Design review of the part built by this model. Coordinates are the model's own, in mm. A direction names the side the tool comes from. Round coordinates to 2 decimals unless told otherwise and drop trailing zeros. Write each loop counter-clockwise with the first axis right and the second up, starting at its lowest first coordinate (ties: lowest second). Pieces come first, ordered by that corner, then holes. Notation, with made-up numbers: M 16.5,-36.5 L 36.5,-36.5 A22 cw 36.5,-19.5 Z; hole C 12,22 d4. An arc over 180 degrees is marked long. One line per question, with ' | ' between items. Start each with the question number.
Item 1: Add section C-C, the plane y = 22.5. State the section outline as (x, z) points (3 decimals), and give its area (3 significant figures).
Item 2: Insertion check: pin 1 Ø6 at (y, z) = (35, 81) entering from -X (3 decimals); pin 2 Ø3 at (x, y) = (17.5, -11) entering from -Z; pin 3 Ø3 at (y, z) = (4.5, 4) entering from -X (3 decimals); pin 4 Ø4 at (x, z) = (96, 188.5) entering from +Y (3 decimals). Each pin has a flat end and moves straight along its axis. Give the tip position at first contact, or say it passes through.
Item 3: Draft analysis for pull direction Z (two halves, no side actions). For faces 5 (the face through (-4, -2, 82.55)), 6 (the face through (-4, -9.525, 251)), 7 (the face through (-2, 1, 0)), 8 (the face through (-48.317, 31.527, 170.739)), state which applies: released by +Z, released by -Z, zero draft, split by the parting line, or undercut.
Item 4: For L1, parallel to Z at x = 95, y = -74; L2, parallel to Y at x = -180.5, z = 269 (3 decimals); L3, parallel to Y at x = -31.5, z = 218 (3 decimals), list the stretches that pass through material, from the lowest coordinate up.
Item 5: Add section D-D, the plane x = 32.5. State the section outline as (y, z) points (3 decimals).
Item 6: Machinability: for faces 1 (the face through (-15.875, 36, 63)), 2 (the face through (-11.891, 20.076, 62.7)), 3 (the face through (11.674, 19.859, 62.7)), 4 (the face through (49.438, 30.884, 170.739)), which of the approach directions +Z, -Z, +X, -X, +Y, -Y give a long, thin tool a straight path to every point of the face, cutting with its end or side? Answer none if there is none.
Item 7: Add section B-B, the plane x = 146. State the section outline as (y, z) points (3 decimals).
Item 8: Add section A-A, the plane z = 171. State the section outline as (x, y) points (3 decimals), and give its area (3 significant figures).
```python
from build123d import *

# Parameters (mm, degrees)
F1_DEPTH = 6.35
F3_DEPTH = 114.3
F5_DEPTH = 101.6
F7_DEPTH = 20.32
F8_W     = 527.05
F8_H     = 295.275
F9_DEPTH = 2.54


with BuildPart() as f1:
    # F0 (on Top) → F1 (new body)
    with BuildSketch(Plane.XY):
        with BuildLine():
            Line((-114.3, -98.425), (114.3, -98.425))
            ThreePointArc((114.3, -98.425), (121.0351920908, -95.6351920908), (123.825, -88.9))
            Line((123.825, -88.9), (123.825, 88.9))
            ThreePointArc((123.825, 88.9), (121.0351920908, 95.6351920908), (114.3, 98.425))
            Line((114.3, 98.425), (-114.3, 98.425))
            ThreePointArc((-114.3, 98.425), (-121.0351920908, 95.6351920908), (-123.825, 88.9))
            Line((-123.825, 88.9), (-123.825, -88.9))
            ThreePointArc((-123.825, -88.9), (-121.0351920908, -95.6351920908), (-114.3, -98.425))
        make_face()
    extrude(amount=F1_DEPTH)

    # F2 (on face) → F3 (join)
    with BuildSketch(Plane.XY.offset(6.35)):
        with BuildLine():
            Line((-1.905, 15.875), (1.905, 15.875))
            ThreePointArc((1.905, 15.875), (11.7832817332, 19.9667182668), (15.875, 29.845))
            Line((15.875, 29.845), (15.875, 42.037))
            ThreePointArc((15.875, 42.037), (11.7832817332, 51.9152817332), (1.905, 56.007))
            Line((1.905, 56.007), (-1.905, 56.007))
            ThreePointArc((-1.905, 56.007), (-11.7832817332, 51.9152817332), (-15.875, 42.037))
            Line((-15.875, 42.037), (-15.875, 29.845))
            ThreePointArc((-15.875, 29.845), (-11.7832817332, 19.9667182668), (-1.905, 15.875))
        make_face()
    extrude(amount=F3_DEPTH)

    # F4 (on face) → F5 (join)
    with BuildSketch(Plane.XY.offset(120.65)):
        with BuildLine():
            ThreePointArc((-15.875, 42.037), (-13.9930859093, 49.0397908043), (-8.8543730782, 54.1558742802))
            Line((-8.8543730782, 54.1558742802), (-88.9, 8.255))
            Line((-88.9, 8.255), (88.9, 8.255))
            Line((88.9, 8.255), (8.8543730782, 54.1558742802))
            ThreePointArc((8.8543730782, 54.1558742802), (13.9930859093, 49.0397908043), (15.875, 42.037))
            Line((15.875, 42.037), (15.875, 29.845))
            ThreePointArc((15.875, 29.845), (11.7832817332, 19.9667182668), (1.905, 15.875))
            Line((1.905, 15.875), (-1.905, 15.875))
            ThreePointArc((-1.905, 15.875), (-11.7832817332, 19.9667182668), (-15.875, 29.845))
            Line((-15.875, 29.845), (-15.875, 42.037))
        make_face()
        with BuildLine():
            ThreePointArc((-1.905, 56.007), (-5.5008466531, 55.536288383), (-8.8543730782, 54.1558742802))
            ThreePointArc((-8.8543730782, 54.1558742802), (-13.9930859093, 49.0397908043), (-15.875, 42.037))
            Line((-15.875, 42.037), (-15.875, 29.845))
            ThreePointArc((-15.875, 29.845), (-11.7832817332, 19.9667182668), (-1.905, 15.875))
            Line((-1.905, 15.875), (1.905, 15.875))
            ThreePointArc((1.905, 15.875), (11.7832817332, 19.9667182668), (15.875, 29.845))
            Line((15.875, 29.845), (15.875, 42.037))
            ThreePointArc((15.875, 42.037), (13.9930859093, 49.0397908043), (8.8543730782, 54.1558742802))
            ThreePointArc((8.8543730782, 54.1558742802), (5.5008466531, 55.536288383), (1.905, 56.007))
            Line((1.905, 56.007), (-1.905, 56.007))
        make_face()
    extrude(amount=F5_DEPTH)

    # F6 (on face) → F7 (join)
    with BuildSketch(Plane.XZ.offset(-8.255)):
        with BuildLine():
            Line((263.525, 406.4), (-263.525, 406.4))
            ThreePointArc((-263.525, 406.4), (-270.2601920908, 403.6101920908), (-273.05, 396.875))
            Line((-273.05, 396.875), (-273.05, 92.075))
            ThreePointArc((-273.05, 92.075), (-270.2601920908, 85.3398079092), (-263.525, 82.55))
            Line((-263.525, 82.55), (263.525, 82.55))
            ThreePointArc((263.525, 82.55), (270.2601920908, 85.3398079092), (273.05, 92.075))
            Line((273.05, 92.075), (273.05, 396.875))
            ThreePointArc((273.05, 396.875), (270.2601920908, 403.6101920908), (263.525, 406.4))
        make_face()
    extrude(amount=F7_DEPTH)

    # F8 (on face) → F9 (cut)
    with BuildSketch(Plane.XZ.offset(12.065)):
        with Locations((0, 249.2375)):
            Rectangle(F8_W, F8_H)
    extrude(amount=-F9_DEPTH, mode=Mode.SUBTRACT)


solid = f1.part
```
Computed values:
1) outline: M -123.825,0 L 123.825,0 L 123.825,6.35 L 13.788,6.35 L 13.788,120.65 L 64.058,120.65 L 64.058,222.25 L -64.058,222.25 L -64.058,120.65 L -13.788,120.65 L -13.788,6.35 L -123.825,6.35 Z | area: 17,700 mm^2
2) pin 1: stops at x = -15.875 | pin 2: stops at z = 0 | pin 3: stops at x = -123.825 | pin 4: stops at y = 8.255
3) face 5: undercut | face 6: undercut | face 7: released by -Z | face 8: zero draft
4) L1: z = 0 to 6.35 | L2: y = -9.525 to 8.255 | L3: y = -9.525 to 41.17
5) outline: M -98.425,0 L 98.425,0 L 98.425,6.35 L -98.425,6.35 Z; M -12.065,82.55 L 8.255,82.55 L 8.255,120.65 L 40.597,120.65 L 40.597,222.25 L 8.255,222.25 L 8.255,406.4 L -12.065,406.4 L -12.065,396.875 L -9.525,396.875 L -9.525,101.6 L -12.065,101.6 Z
6) face 1: -X, +Y | face 2: -X | face 3: +X | face 4: +Z, +X, +Y
7) outline: M -12.065,82.55 L 8.255,82.55 L 8.255,406.4 L -12.065,406.4 L -12.065,396.875 L -9.525,396.875 L -9.525,101.6 L -12.065,101.6 Z
8) outline: M -273.05,-12.065 L -263.525,-12.065 L -263.525,-9.525 L 263.525,-9.525 L 263.525,-12.065 L 273.05,-12.065 L 273.05,8.255 L 88.9,8.255 L 8.854,54.156 A13.97 ccw 1.905,56.007 L -1.905,56.007 A13.97 ccw -8.854,54.156 L -88.9,8.255 L -273.05,8.255 Z | area: 14,300 mm^2
